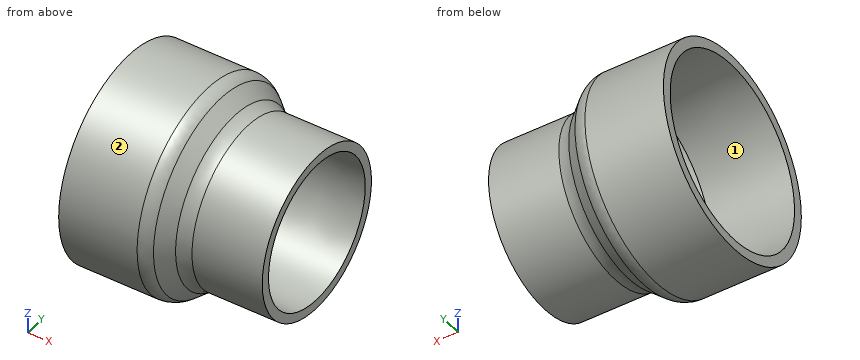
```python
from build123d import *

# Parameters (mm, degrees)
FILLET1_R = 12.7


with BuildPart() as part:
    # Sketch1 → Revolve1 (revolve)
    with BuildSketch(Plane.XY):
        Polygon((-7.2517, -57.0357), (7.80462683, -44.40194171), (7.7597, -44.3484), (58.5597, -44.6532), (58.5597, -50.3682), (10.434859531, -50.3682), (-5.381498273, -63.6397), (-58.5597, -63.6397), (-58.5597, -57.3786), align=None)
    revolve(axis=Axis((-58.5597, 0, 0), (1, 0, 0)))

    # Fillet1
    fillet1_edges = [part.edges().sort_by_distance(p)[0] for p in [
        (-5.381498273, 63.6397, 0),
        (10.434859531, 50.3682, 0),
    ]]
    fillet(fillet1_edges, radius=FILLET1_R)


solid = part.part
```
Model file for the job. Use its own axes, mm. Face numbers are marked on the shaded views. Give positions to 0.01 mm unless a question says otherwise; leave off trailing zeros. Write each loop counter-clockwise with the first axis right and the second up, starting at its lowest first coordinate (ties: lowest second). Pieces come first, ordered by that corner, then holes. Notation, with made-up numbers: M 24,-5 L 44,-5 A25 ccw 44,18 Z; hole C -4.5,17.25 d8. An arc over 180 degrees is marked long. Use a Markdown table: item, result.
1) Drill centre lines: line 1 (Y direction, x = 30, z = -33.5); line 2 (Z direction, x = 14, y = 24.5); line 3 (Z direction, x = -26, y = -29). Where is each one in solid material? Low to high. Write a range as from..to.
Responses:
| item | result |
|---|---|
| line 1 | y = -37.61..-29.26, 29.26..37.61 |
| line 2 | z = -44.06..-37.01, 37.01..44.06 |
| line 3 | z = -56.65..-49.26, 49.26..56.65 |
2) Cut at B-B (x = -47). List the corners of the cut face in (y, z), and give its area (3 significant figures).
Responses:
| item | result |
|---|---|
| outline | C 0,0 d127.28; hole C 0,0 d114.6 |
| area | 2,410 mm2 |
3) Pin check, flat tips, straight feed: pin 1 (4 mm diameter, centred on x = -32.5, y = 17, fed in from -Z); pin 2 (8 mm diameter, centred on x = 26.5, y = 2, fed in from +Z); pin 3 (2 mm diameter, centred on x = -21.5, y = -28, fed in from +Z). Stop position of each tip, or through.
Responses:
| item | result |
|---|---|
| pin 1 | stops at z = -61.85 |
| pin 2 | stops at z = 50.37 |
| pin 3 | stops at z = 57.63 |
4) Cut at A-A (x = 18). List the corners of the cut face in (y, z), and give its area (3 significant figures).
Responses:
| item | result |
|---|---|
| outline | C 0,0 d100.74; hole C 0,0 d88.82 |
| area | 1,770 mm2 |
5) Pull direction Z, two halves, no side cores. Call the marked faces 1 and 2: +Z half, -Z half, draft (parallel to the pull), parting line (faces both ways), or undercut.
Responses:
| item | result |
|---|---|
| face 1 | undercut |
| face 2 | parting line |
